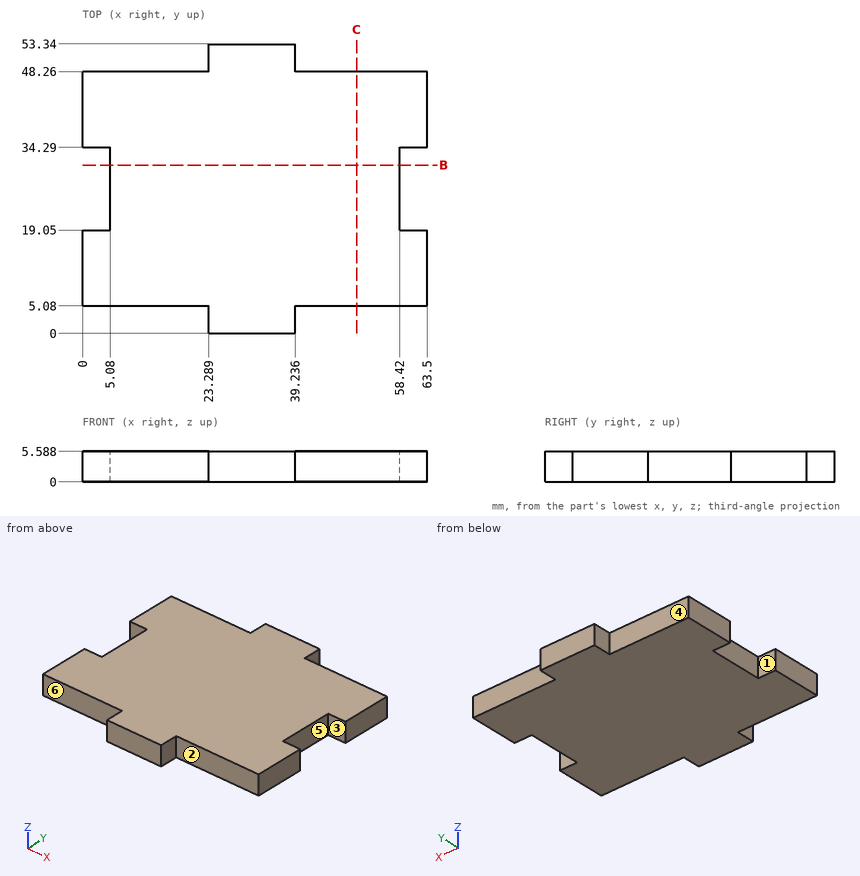
Source: three-view drawing plus pictorial views. Frame: mm from the lowest corner of the part. A direction names the side the tool comes from. Give positions to 0.01 mm unless a question says otherwise; leave off trailing zeros. Order: outer loops, then holes, each group sorted by start corner. A loop starts at its lowest first (then second) coordinate and runs counter-clockwise, first axis right, second up. Notation, with made-up numbers: (31.5, 35.25) -> (45.5, 35.25) arc R21 ccw to (45.5, 67.25) -> close; hole circle Ø9 at (-27, -33.75). An arc over 180 degrees is marked (long way). Use a Markdown table: item, result.
Q1. Section C-C (x = 50.5). Return the cut outline in (y, z).
A:
| item | result |
|---|---|
| outline | (5.08, 0) -> (48.26, 0) -> (48.26, 5.59) -> (5.08, 5.59) -> close |
Q2. Material intervals for line 1 (Y direction, x = 60.5, z = 0.5); line 2 (Y direction, x = 44, z = 1.1); line 3 (X direction, y = 30.5, z = 0.45), sorted ascending. Write a range as [from, to].
A:
| item | result |
|---|---|
| line 1 | [5.08, 19.05], [34.29, 48.26] |
| line 2 | [5.08, 48.26] |
| line 3 | [5.08, 58.42] |
Q3. First-contact query: P1, Ø1.7, axis at x = 16, z = 2, coming from the +Y side; P2, Ø1.5, axis at y = 50, z = 3, coming from the -X side; P3, Ø1.7, axis at x = 13.5, z = 3, coming from the -Y side; P4, Ø12, axis at x = 28.5, y = 40, coming from the -Z side. Flat tips, straight axial feed; report the tip coordinate or a pass-through.
A:
| item | result |
|---|---|
| P1 | y = 48.26 |
| P2 | x = 23.29 |
| P3 | y = 5.08 |
| P4 | z = 0 |
Q4. Pull-direction query (Y, two-part tool) for the marked faces 4, 5 and 6; classes: +Y half, -Y half, draft (parallel to the pull), parting line (faces both ways), or undercut.
A:
| item | result |
|---|---|
| face 4 | +Y half |
| face 5 | undercut |
| face 6 | -Y half |
Q5. Section B-B (y = 31). Return the cut outline in (x, z), and give its area (3 significant figures).
A:
| item | result |
|---|---|
| outline | (5.08, 0) -> (58.42, 0) -> (58.42, 5.59) -> (5.08, 5.59) -> close |
| area | 298 mm^2 |
Q6. Access query for the marked faces 1, 2 and 3. Directions: +Z, -Z, +X, -X, +Y, -Y. A direction counts if a zero-diameter tool reaches every point of the face in a straight line with its end or side. Return the directions, or none.
A:
| item | result |
|---|---|
| face 1 | +Z, -Z, -X |
| face 2 | +Z, -Z, +X, -Y |
| face 3 | +Z, -Z, +X |
